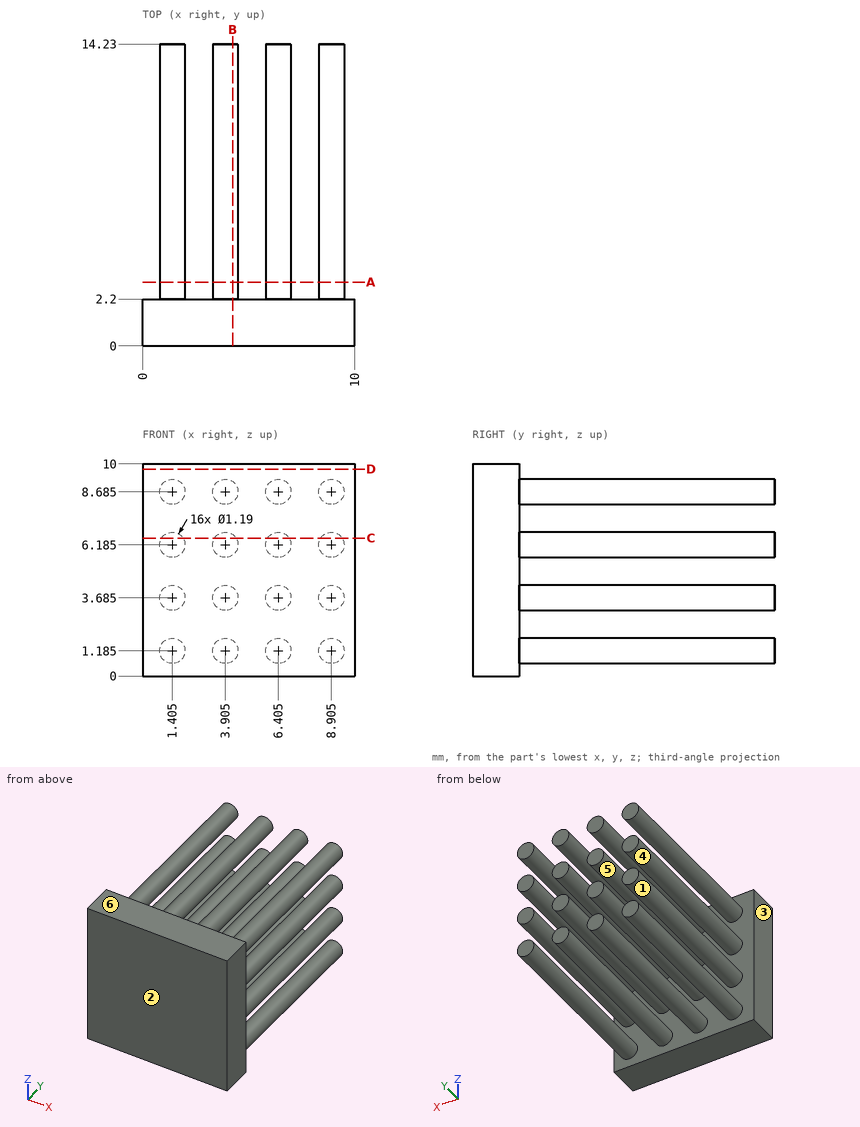
Print and shaded views of the part. All mm, measured from the part's lowest x, y and z. A direction names the side the tool comes from. Coordinates: 2 decimals unless noted, no trailing zeros. Write each loop counter-clockwise with the first axis right and the second up, starting at its lowest first coordinate (ties: lowest second). Pieces come first, ordered by that corner, then holes.
(1) Cut at C-C, the plane z = 6.5. List the corners of the cut face in (x, y), and give its area (3 significant figures).
(2) Cut at B-B, the plane x = 4.25. List the corners of the cut face in (y, z).
(3) 3-axis set-ups, long thin cutter, end or side, ignore diameter. For the marked faces 1 and 2: which of +Z, -Z, +X, -X, +Y, -Y reach the whole face in a straight line?
(4) Cut at D-D, the plane z = 9.75. List the corners of the cut face in (x, y), and give its area (3 significant figures).
(5) Two-plate mould, pull along Z, no slides. Class the marked faces 3, 4, 5 and 6: +Z half, -Z half, draft (parallel to the pull), parting line (faces both ways), or undercut.
(6) Drill centre lines: probe 1 along X at (y, z) = (6, 3.75); probe 2 along Z at (x, y) = (4, 13.25); probe 3 along Z at (x, y) = (1.75, 9.5). Where is each one in solid material? Low to high.
(7) Flat gauge pins, fed straight in: pin 1 (1.5 mm diameter, centred on x = 3, y = 11, fed in from +Z); pin 2 (3 mm diameter, centred on x = 8, z = 6.5, fed in from +Y); pin 3 (1 mm diameter, centred on y = 6, z = 4.5, fed in from +X); pin 4 (1.5 mm diameter, centred on x = 6, y = 10, fed in from -Z). Where does each tip first touch, or does it go through?
(8) Cut at A-A, the plane y = 3. Count the separate pieces of the cut face and the enclosed holes in it, and give its area (3 significant figures).
Geometry says:
1. outline: (0, 0) - (10, 0) - (10, 2.2) - (9.41, 2.2) - (9.41, 14.23) - (8.4, 14.23) - (8.4, 2.2) - (6.91, 2.2) - (6.91, 14.23) - (5.9, 14.23) - (5.9, 2.2) - (4.41, 2.2) - (4.41, 14.23) - (3.4, 14.23) - (3.4, 2.2) - (1.91, 2.2) - (1.91, 14.23) - (0.9, 14.23) - (0.9, 2.2) - (0, 2.2) - close
1. area: 70.6 mm2
2. outline: (0, 0) - (2.2, 0) - (2.2, 0.7) - (14.23, 0.7) - (14.23, 1.67) - (2.2, 1.67) - (2.2, 3.2) - (14.23, 3.2) - (14.23, 4.17) - (2.2, 4.17) - (2.2, 5.7) - (14.23, 5.7) - (14.23, 6.67) - (2.2, 6.67) - (2.2, 8.2) - (14.23, 8.2) - (14.23, 9.17) - (2.2, 9.17) - (2.2, 10) - (0, 10) - close
3. face 1: +Y
3. face 2: +Z, -Z, +X, -X, -Y
4. outline: (0, 0) - (10, 0) - (10, 2.2) - (0, 2.2) - close
4. area: 22.0 mm2
5. face 3: draft
5. face 4: undercut
5. face 5: undercut
5. face 6: +Z half
6. probe 1: x = 0.81 to 2, 3.31 to 4.5, 5.81 to 7, 8.31 to 9.5
6. probe 2: z = 0.6 to 1.77, 3.1 to 4.27, 5.6 to 6.77, 8.1 to 9.27
6. probe 3: z = 0.7 to 1.67, 3.2 to 4.17, 5.7 to 6.67, 8.2 to 9.17
7. pin 1: stops at z = 9.26
7. pin 2: stops at y = 14.23
7. pin 3: stops at x = 9.41
7. pin 4: stops at z = 0.59
8. separate pieces: 16
8. enclosed holes: 0
8. area: 17.8 mm2
